```python
from build123d import *

# Parameters (mm, degrees)
SKETCH1_W           = 105
SKETCH1_H           = 105
BOSS_EXTRUDE1_DEPTH = 12
SKETCH2_R           = 22
BOSS_EXTRUDE2_DEPTH = 98
BOSS_EXTRUDE3_START = -82
BOSS_EXTRUDE3_DEPTH = 82
HOLE1_D             = 25
HOLE2_REACH         = 146.439
HOLE2_BORE_R        = 6
BOSS_EXTRUDE4_START = -76
BOSS_EXTRUDE4_DEPTH = 76
HOLE3_REACH         = 150.312
HOLE3_BORE_R        = 5
FILLET1_R           = 10
HOLE4_D             = 10
HOLE4_CBORE_D       = 18
HOLE4_CBORE_DEPTH   = 2


with BuildPart() as part:
    # Sketch1 → Boss-Extrude1 (new body)
    with BuildSketch(Plane.XY):
        Rectangle(SKETCH1_W, SKETCH1_H)
    extrude(amount=BOSS_EXTRUDE1_DEPTH)

    # Sketch2 → Boss-Extrude2 (add)
    with BuildSketch(Plane.XY.offset(12)):
        Circle(SKETCH2_R)
    extrude(amount=BOSS_EXTRUDE2_DEPTH)

    # Sketch3 → Boss-Extrude3 (add)
    with BuildSketch(Plane.XY.offset(110).offset(BOSS_EXTRUDE3_START)):
        with BuildLine():
            Line((-15, 16.093476939), (-15, 25))
            Line((-15, 25), (15, 25))
            Line((15, 25), (15, 16.093476939))
            ThreePointArc((15, 16.093476939), (0, 22), (-15, 16.093476939))
        make_face()
    extrude(amount=BOSS_EXTRUDE3_DEPTH)

    # Hole1 (through all)
    with Locations(Plane.XY.offset(110)):
        with Locations((0, 0)):
            Hole(HOLE1_D / 2)

    # Hole2 bore → Hole2 (cut, up to next)
    with BuildSketch(Plane(origin=(0, 25, 0), x_dir=(1, 0, 0), z_dir=(0, 1, 0)), mode=Mode.PRIVATE) as hole2_sk1:
        with Locations((0, -40.5)):
            Circle(HOLE2_BORE_R)
    hole2_tool1 = extrude(hole2_sk1.sketch, amount=-HOLE2_REACH, mode=Mode.PRIVATE) & part.part
    # Hole2 bore → Hole2 (cut, up to next)
    with BuildSketch(Plane(origin=(0, 25, 0), x_dir=(1, 0, 0), z_dir=(0, 1, 0)), mode=Mode.PRIVATE) as hole2_sk2:
        with Locations((0, -97.5)):
            Circle(HOLE2_BORE_R)
    hole2_tool2 = extrude(hole2_sk2.sketch, amount=-HOLE2_REACH, mode=Mode.PRIVATE) & part.part
    add(hole2_tool1.solids().sort_by_distance((0, 25, 40.5))[0], mode=Mode.SUBTRACT)
    add(hole2_tool2.solids().sort_by_distance((0, 25, 97.5))[0], mode=Mode.SUBTRACT)

    # Sketch9 → Boss-Extrude4 (add)
    with BuildSketch(Plane.XY.offset(110).offset(BOSS_EXTRUDE4_START)):
        with BuildLine():
            Line((0, -22), (32, -22))
            Line((32, -22), (32, 8))
            Line((32, 8), (20.493901532, 8))
            ThreePointArc((20.493901532, 8), (18.165902125, -12.409673646), (0, -22))
        make_face()
    extrude(amount=BOSS_EXTRUDE4_DEPTH)

    # Hole3 bore → Hole3 (cut, up to next)
    with BuildSketch(Plane(origin=(32, 0, 0), x_dir=(0, 0, -1), z_dir=(1, 0, 0)), mode=Mode.PRIVATE) as hole3_sk1:
        with Locations((-81.5, -7)):
            Circle(HOLE3_BORE_R)
    hole3_tool1 = extrude(hole3_sk1.sketch, amount=-HOLE3_REACH, mode=Mode.PRIVATE) & part.part
    # Hole3 bore → Hole3 (cut, up to next)
    with BuildSketch(Plane(origin=(32, 0, 0), x_dir=(0, 0, -1), z_dir=(1, 0, 0)), mode=Mode.PRIVATE) as hole3_sk2:
        with Locations((-56.5, -7)):
            Circle(HOLE3_BORE_R)
    hole3_tool2 = extrude(hole3_sk2.sketch, amount=-HOLE3_REACH, mode=Mode.PRIVATE) & part.part
    add(hole3_tool1.solids().sort_by_distance((32, -7, 81.5))[0], mode=Mode.SUBTRACT)
    add(hole3_tool2.solids().sort_by_distance((32, -7, 56.5))[0], mode=Mode.SUBTRACT)

    # Fillet1
    fillet1_edges = [part.edges().sort_by_distance(p)[0] for p in [
        (52.5, -52.5, 6),
        (-52.5, -52.5, 6),
        (-52.5, 52.5, 6),
        (52.5, 52.5, 6),
    ]]
    fillet(fillet1_edges, radius=FILLET1_R)

    # Hole4 (through all)
    with Locations(Plane.XY.offset(12)):
        with Locations((42.5, -42.5), (42.5, 42.5), (-42.5, 42.5), (-42.5, -42.5)):
            CounterBoreHole(HOLE4_D / 2, HOLE4_CBORE_D / 2, HOLE4_CBORE_DEPTH)


solid = part.part
```
For this review, take the finished solid that the model builds, in its own axes (mm). A direction names the side the tool comes from. Round coordinates to 2 decimals unless told otherwise and drop trailing zeros. Write each loop counter-clockwise with the first axis right and the second up, starting at its lowest first coordinate (ties: lowest second). Pieces come first, ordered by that corner, then holes. Notation, with made-up numbers: (14.5, 25.25) -> (26.5, 25.25) arc R29 ccw to (26.5, 54.25) -> close; hole circle Ø8 at (34.25, 13.5). An arc over 180 degrees is marked (long way). Use one line per item in the form item = value.
Q1. Consider section D-D (z = 40.5). State the section outline as (x, y) points, then the cut area to 3 significant figures.
Resolved:
outline = (-15, 16.09) arc R22 ccw to (0, -22) -> (32, -22) -> (32, 8) -> (20.49, 8) arc R22 ccw to (15, 16.09) -> (15, 25) -> (6, 25) -> (6, 10.97) arc R12.5 cw (long way) to (-6, 10.97) -> (-6, 25) -> (-15, 25) -> close
area = 1,430 mm²
Q2. To check wall thickness, follow probe 1 along Y at (x, z) = (-42, 7); probe 2 along Y at (x, z) = (42.5, 11.15). State the ranges of each line that lie inside material, in increasing order. Write a range as from..to.
Resolved:
probe_1 = -52.5..-47.47, -37.53..37.53, 47.47..52.5
probe_2 = -52.5..-51.5, -33.5..33.5, 51.5..52.5
Q3. Consider section B-B (z = 64.5). State the section outline as (x, y) points.
Resolved:
outline = (-15, 16.09) arc R22 ccw to (0, -22) -> (32, -22) -> (32, 8) -> (20.49, 8) arc R22 ccw to (15, 16.09) -> (15, 25) -> (-15, 25) -> close; hole circle Ø25 at (0, 0)
Q4. Consider section A-A (y = 0). State the section outline as (x, z) points.
Resolved:
outline = (-52.5, 0) -> (-12.5, 0) -> (-12.5, 110) -> (-22, 110) -> (-22, 12) -> (-52.5, 12) -> close; (12.5, 0) -> (52.5, 0) -> (52.5, 12) -> (22, 12) -> (22, 34) -> (32, 34) -> (32, 110) -> (12.5, 110) -> close
Q5. Consider section C-C (x = 46). State the section outline as (y, z) points.
Resolved:
outline = (-51.87, 0) -> (-46.07, 0) -> (-46.07, 10) -> (-50.79, 10) -> (-50.79, 12) -> (-51.87, 12) -> close; (-38.93, 0) -> (38.93, 0) -> (38.93, 10) -> (34.21, 10) -> (34.21, 12) -> (-34.21, 12) -> (-34.21, 10) -> (-38.93, 10) -> close; (46.07, 0) -> (51.87, 0) -> (51.87, 12) -> (50.79, 12) -> (50.79, 10) -> (46.07, 10) -> close
Q6. Machinability: for faces 4 (the cylindrical face through (-38.815, -39.121, 4.93)), 5 (the cylindrical face through (-49.133, -36.417, 11.014)), 6 (the cylindrical face through (-5.994, 18.081, 40.236)), 7 (the cylindrical face through (21.11, -11.88, 57.58)), 8 (the flat face through (-1, 52.5, 6)), which of the approach directions +Z, -Z, +X, -X, +Y, -Y give a long, thin tool a straight path to every point of the face, cutting with its end or side? Answer none if there is none.
Resolved:
face_4 = +Z, -Z
face_5 = +Z
face_6 = +Y
face_7 = +X
face_8 = +Z, -Z, +X, -X, +Y
Q7. The part is to be moulded in two halves that separate along X. For faces 1 (the cylindrical face through (-5.994, 18.081, 97.236)), 2 (the flat face through (16, -22, 71)), 3 (the flat face through (-15, 20, 68)), say which applies: released by +X, released by -X, zero draft, split by the parting line, or undercut.
Resolved:
face_1 = undercut
face_2 = zero draft
face_3 = released by -X
Q8. Clearance check with flat-ended pins moving along their axes: pin 1 Ø15.5 at (x, z) = (0, 97.5) entering from +Y; pin 2 Ø2.5 at (y, z) = (20, 67) entering from -X; pin 3 Ø1.5 at (y, z) = (24, 40.5) entering from +X. State where each tip first meets the part, or that it passes through.
Resolved:
pin_1 = 25
pin_2 = -15
pin_3 = 15
